The model under review builds one solid part; all positions refer to its coordinate system, in mm. Coordinates: 2 decimals unless noted, no trailing zeros. Order: outer loops, then holes, each group sorted by start corner. A loop starts at its lowest first (then second) coordinate and runs counter-clockwise, first axis right, second up. Notation, with made-up numbers: M 3,72.5 L 60,72.5 A34 cw 60,106.5 Z; hole C 38.5,81 d9. An arc over 180 degrees is marked long. One line per item, written item: value.
```python
from build123d import *

# Parameters (mm, degrees)
BOSS_EXTRUDE1_DEPTH = 6.35
SKETCH15_R          = 5.715
CUT_EXTRUDE1_DEPTH  = 65.027197676


with BuildPart() as part:
    # Sketch13 → Boss-Extrude1 (new body)
    with BuildSketch(Plane.XY):
        with BuildLine():
            Line((-34.961025172, 28.467243349), (-9.847867764, 8.991202672))
            ThreePointArc((-9.847867764, 8.991202672), (4.12074162, 12.682338645), (13.251988711, 1.485604323))
            Line((13.251988711, 1.485604323), (45.016689319, 2.480908651))
            ThreePointArc((45.016689319, 2.480908651), (13.932031191, 42.878383037), (-34.961025172, 28.467243349))
        make_face()
    extrude(amount=BOSS_EXTRUDE1_DEPTH)

    # Sketch15 → Cut-Extrude1 (cut, through all)
    with BuildSketch(Plane.XY.offset(6.35)):
        with BuildLine():
            ThreePointArc((-15.475292944, 13.355447276), (-17.389315258, 19.694740336), (-24.005496972, 19.970887857))
            Line((-24.005496972, 19.970887857), (-15.475292944, 13.355447276))
        make_face()
        with Locations((7.979904528, 24.559620794)):
            Circle(SKETCH15_R)
        with BuildLine():
            ThreePointArc((31.159448366, 2.046710575), (25.644529482, 5.712196576), (20.369909931, 1.708634847))
            Line((20.369909931, 1.708634847), (31.159448366, 2.046710575))
        make_face()
    extrude(amount=-CUT_EXTRUDE1_DEPTH, mode=Mode.SUBTRACT)


solid = part.part
```
(1) We need section A-A, the plane y = 11.5. State the section outline as (x, z) points, plus the area to 3 significant figures.
Geometry results:
outline: M -13.08,0 L -6.75,0 L -6.75,6.35 L -13.08,6.35 Z; M 6.75,0 L 43.59,0 L 43.59,6.35 L 6.75,6.35 Z
area: 274 mm2
(2) We need section D-D, the plane x = 33. State the section outline as (y, z) points.
Geometry results:
outline: M 2.1,0 L 30.72,0 L 30.72,6.35 L 2.1,6.35 Z
(3) Insertion check: pin 1 Ø2 at (y, z) = (6, 1) entering from -X; pin 2 Ø1.5 at (y, z) = (19, 3.5) entering from +X; pin 3 Ø1 at (x, z) = (2.5, 5) entering from -Y. Each pin has a flat end and moves straight along its axis. Give the tip position at first contact, or say it passes through.
Geometry results:
pin 1: stops at x = 11.35
pin 2: stops at x = 41.23
pin 3: stops at y = 12.99
(4) Mouldability with a two-part tool opening along Y and no side actions: class faces 1 (the flat face through (-29.56, 24.28, 3.13)), 2 (the cylindrical face through (-17.31, 19.63, 3.22)), 3 (the cylindrical face through (6.74, 18.98, 3.22)), 4 (the flat face through (4, 19, 6.35)) as +Y half, -Y half, draft (parallel to the pull), parting line (faces both ways), or undercut.
Geometry results:
face 1: -Y half
face 2: undercut
face 3: undercut
face 4: draft
(5) For L1, parallel to X at y = 21, z = 0.5; L2, parallel to Y at x = 3, z = 1; L3, parallel to X at y = 21.5, z = 6, list the stretches that pass through material, from the lowest coordinate up.
Geometry results:
L1: x = -25.33 to 3.51, 12.45 to 39.9
L2: y = 12.99 to 21.76, 27.36 to 44.99
L3: x = -25.98 to 3.15, 12.81 to 39.63
(6) We need section C-C, the plane y = 25.5. State the section outline as (x, z) points, plus the area to 3 significant figures.
Geometry results:
outline: M -31.13,0 L 2.34,0 L 2.34,6.35 L -31.13,6.35 Z; M 13.62,0 L 37.18,0 L 37.18,6.35 L 13.62,6.35 Z
area: 362 mm2
(7) We need section B-B, the plane z = 1.5. State the section outline as (x, y) points (1 decimal).
Geometry results:
outline: M -35,28.5 L -24,20 A5.7 cw -15.5,13.4 L -9.8,9 A13.3 cw 13.3,1.5 L 20.4,1.7 A5.7 cw 31.2,2 L 45,2.5 A45.1 ccw Z; hole C 8,24.6 d11.4
